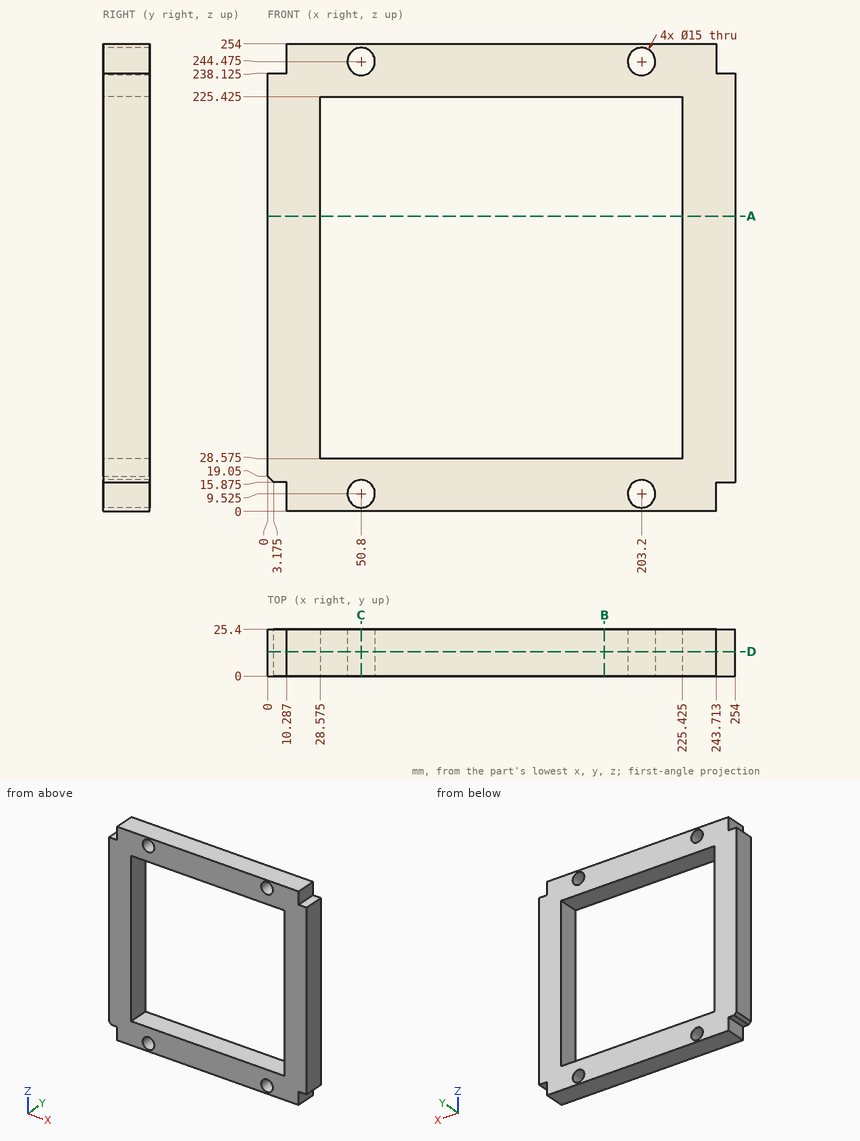
Design review of the part shown in the three views and the two pictorial views. Dimensions are in mm from the part's minimum x, y and z. Round coordinates to 2 decimals unless told otherwise and drop trailing zeros. Order: outer loops, then holes, each group sorted by start corner. A loop starts at its lowest first (then second) coordinate and runs counter-clockwise, first axis right, second up. Notation, with made-up numbers: M -32,60 L 12,60 A18 ccw 12,92 Z; hole C 54.5,-8.5 d11. An arc over 180 degrees is marked long. Put each result on its own line as item: value.
Q1. Insertion check: pin 1 Ø12.5 at (x, y) = (87, 13) entering from -Z; pin 2 Ø13.5 at (x, z) = (50.8, 244.475) entering from +Y (3 decimals); pin 3 Ø12.5 at (y, z) = (6.5, 6) entering from +X; pin 4 Ø8 at (y, z) = (12, 10) entering from -X. Each pin has a flat end and moves straight along its axis. Give the tip position at first contact, or say it passes through.
Reported:
pin 1: z = 0
pin 2: through
pin 3: x = 243.71
pin 4: x = 10.29
Q2. Consider section A-A (z = 160.5). State the section outline as (x, y) points (3 decimals).
Reported:
outline: M 0,0 L 28.575,0 L 28.575,25.4 L 0,25.4 Z; M 225.425,0 L 254,0 L 254,25.4 L 225.425,25.4 Z
Q3. Consider section B-B (x = 183). State the section outline as (y, z) points (3 decimals), and give its area (3 significant figures).
Reported:
outline: M 0,0 L 25.4,0 L 25.4,28.575 L 0,28.575 Z; M 0,225.425 L 25.4,225.425 L 25.4,254 L 0,254 Z
area: 1,450 mm²
Q4. Consider section D-D (y = 13.25). State the section outline as (x, z) points (3 decimals), and give its area (3 significant figures).
Reported:
outline: M 0,19.05 L 3.175,15.875 L 10.287,15.875 L 10.287,0 L 243.713,0 L 243.713,15.875 L 254,15.875 L 254,238.125 L 243.713,238.125 L 243.713,254 L 10.287,254 L 10.287,238.125 L 0,238.125 Z; hole M 28.575,28.575 L 225.425,28.575 L 225.425,225.425 L 28.575,225.425 Z; hole C 50.8,9.525 d15; hole C 50.8,244.475 d15; hole C 203.2,9.525 d15; hole C 203.2,244.475 d15
area: 24,400 mm²
Q5. To check wall thickness, follow line 1 (Z direction, x = 50.8, y = 18.5) (3 decimals); line 2 (Z direction, x = 160.5, y = 6) (3 decimals). State the ranges of each line that lie inside material, in increasing order.
Reported:
line 1: 0 to 2.025, 17.025 to 28.575, 225.425 to 236.975, 251.975 to 254
line 2: 0 to 28.575, 225.425 to 254
Q6. Consider section C-C (x = 50.8). State the section outline as (y, z) points (3 decimals), and give its area (3 significant figures).
Reported:
outline: M 0,0 L 25.4,0 L 25.4,2.025 L 0,2.025 Z; M 0,17.025 L 25.4,17.025 L 25.4,28.575 L 0,28.575 Z; M 0,225.425 L 25.4,225.425 L 25.4,236.975 L 0,236.975 Z; M 0,251.975 L 25.4,251.975 L 25.4,254 L 0,254 Z
area: 690 mm²
